from build123d import *

# Parameters (mm, degrees)
SKETCH1_W                    = 16
SKETCH1_H                    = 15
BOSS_EXTRUDE1_DEPTH          = 0.64
EDGE_FLANGE1_STRIP_W         = 5.12
EDGE_FLANGE1_STRIP_H         = 0.64
EDGE_FLANGE1_STRIP_CUT_DEPTH = 16
EDGE_FLANGE1_DEPTH           = 16
SKETCH9_R                    = 1.9
CUT_EXTRUDE1_DEPTH           = 27.570660511
SKETCH10_R                   = 1.9
CUT_EXTRUDE2_DEPTH           = 27.570660511
CHAMFER1_SIZE                = 5
FILLET1_R                    = 2.5


# Sheet-metal steps are written as plain solids
with BuildPart() as part:
    # Sketch1 → Boss-Extrude1 (new body)
    with BuildSketch(Plane(origin=(0, 0, 0), x_dir=(0, 0, -1), z_dir=(1, 0, 0))):
        with Locations((8, 7.5)):
            Rectangle(SKETCH1_W, SKETCH1_H)
    extrude(amount=BOSS_EXTRUDE1_DEPTH)

    # Edge-Flange1 strip (across the edge) → Edge-Flange1 strip cut (cut)
    with BuildSketch(Plane(origin=(0.64, 15, -16), x_dir=(0, -1, 0), z_dir=(0, 0, 1))):
        with Locations((-0.64, -0.32)):
            Rectangle(EDGE_FLANGE1_STRIP_W, EDGE_FLANGE1_STRIP_H)
    extrude(amount=EDGE_FLANGE1_STRIP_CUT_DEPTH, mode=Mode.SUBTRACT)

    # Edge-Flange1 section (across the edge) → Edge-Flange1 (add)
    with BuildSketch(Plane(origin=(0.64, 15, -16), x_dir=(0, -1, 0), z_dir=(0, 0, 1))):
        with BuildLine():
            Line((0, 1.28), (0, 14.36))
            Line((0, 14.36), (0.64, 14.36))
            Line((0.64, 14.36), (0.64, 1.28))
            ThreePointArc((0.64, 1.28), (1.01490332, 0.37490332), (1.92, 0))
            Line((1.92, 0), (1.92, -0.64))
            ThreePointArc((1.92, -0.64), (0.56235498, -0.07764502), (0, 1.28))
        make_face()
    extrude(amount=EDGE_FLANGE1_DEPTH)

    # Sketch9 → Cut-Extrude1 (cut, through all)
    with BuildSketch(Plane.ZY):
        with Locations((-12, 5)):
            Circle(SKETCH9_R)
        with Locations((-4, 5)):
            Circle(SKETCH9_R)
    extrude(amount=-CUT_EXTRUDE1_DEPTH, mode=Mode.SUBTRACT)

    # Sketch10 → Cut-Extrude2 (cut, through all)
    with BuildSketch(Plane(origin=(0, 15, 0), x_dir=(1, 0, 0), z_dir=(0, 1, 0))):
        with Locations(Location((10, 8, 0), (0, 0, 180))):
            Circle(SKETCH10_R)
    extrude(amount=-CUT_EXTRUDE2_DEPTH, mode=Mode.SUBTRACT)

    # Chamfer1
    chamfer1_edges = [part.edges().sort_by_distance(p)[0] for p in [
        (15, 14.68, -16),
        (15, 14.68, 0),
    ]]
    chamfer(chamfer1_edges, length=CHAMFER1_SIZE)

    # Fillet1
    fillet1_edges = [part.edges().sort_by_distance(p)[0] for p in [
        (10, 14.68, -16),
        (15, 14.68, -5),
        (15, 14.68, -11),
        (10, 14.68, 0),
        (0.32, 0, 0),
        (0.32, 0, -16),
    ]]
    fillet(fillet1_edges, radius=FILLET1_R)


solid = part.part
Read the model definition and answer for the solid it produces. Units are mm, in the model's axes. A direction names the side the tool comes from. Coordinates: 2 decimals unless noted, no trailing zeros. Loops run counter-clockwise (first coordinate to the right, second up) from the corner with the lowest first, then second, coordinate; pieces in that order, holes last. Notation, with made-up numbers: (21.25, 9.5) -> (36.25, 9.5) arc R17 ccw to (36.25, 39.5) -> close; hole circle Ø7 at (0.25, 2). An arc over 180 degrees is marked (long way). Write item = value, one per line. Start each with the question number.
1) The part is cut by section B-B, the plane z = -12. Determine the outline of the cut face in (x, y), plus the area to 3 significant figures.
2) The part is cut by section D-D, the plane z = -1.75. Determine the outline of the cut face in (x, y).
3) Given P1, Ø5, axis at y = 9, z = -5, coming from the -X side; P2, Ø4, axis at y = 4.5, z = -10, coming from the +X side; P3, Ø6, axis at x = 9, z = -14, coming from the -Y side, each flat-ended and moving along its own axis, determine where each tip first touches the part or whether it passes through.
4) The part is cut by section C-C, the plane x = 8.75. Determine the outline of the cut face in (y, z), plus the area to 3 significant figures.
5) For faces 5 (the face through (0.64, 7, -8)), 6 (the face through (0.2, 10.6, 0)), determine the directions among +Z, -Z, +X, -X, +Y, -Y from which every point of the face is accessible in a straight line to the end or side of a thin tool.
6) The part is cut by section A-A, the plane y = 5. Determine the outline of the cut face in (x, z).
7) Find the intervals of material crossed by L1, parallel to Y at x = 2.25, z = -15; L2, parallel to X at y = 12.5, z = -8; L3, parallel to Y at x = 0.3, z = -4, in increasing order. Write a range as from..to.
8) The mould has two halves that part along Y. Classify faces 1 (the face through (0.316, 6.284, -5.4)), 2 (the face through (0.324, 0.752, -15.287)), 3 (the face through (0.316, 6.602, -10.979)), 4 (the face through (0.2, 10.6, -16)): pulls with the +Y half, pulls with the -Y half, needs draft (parallel to the pull), parting line crosses it, or undercut.
Result:
q1.outline = (0, 0) -> (0.64, 0) -> (0.64, 3.1) -> (0, 3.1) -> close; (0, 6.9) -> (0.64, 6.9) -> (0.64, 13.08) arc R1.28 cw to (1.92, 14.36) -> (14, 14.36) -> (14, 15) -> (1.92, 15) arc R1.92 ccw to (0, 13.08) -> close
q1.area = 15.3 mm²
q2.outline = (0, 0.12) -> (0.64, 0.12) -> (0.64, 13.08) arc R1.28 cw to (1.92, 14.36) -> (11.75, 14.36) -> (11.75, 15) -> (1.92, 15) arc R1.92 ccw to (0, 13.08) -> close
q3.P1 = 0
q3.P2 = 0.64
q3.P3 = 14.36
q4.outline = (14.36, -16) -> (15, -16) -> (15, -9.43) -> (14.36, -9.43) -> close; (14.36, -6.57) -> (15, -6.57) -> (15, 0) -> (14.36, 0) -> close
q4.area = 8.41 mm²
q5.face_5 = +Z, -Z, +X, -Y
q5.face_6 = +Z, +X, -X, +Y, -Y
q6.outline = (0, -16) -> (0.64, -16) -> (0.64, -13.9) -> (0, -13.9) -> close; (0, -10.1) -> (0.64, -10.1) -> (0.64, -5.9) -> (0, -5.9) -> close; (0, -2.1) -> (0.64, -2.1) -> (0.64, 0) -> (0, 0) -> close
q7.L1 = 14.36..15
q7.L2 = 0..0.64
q7.L3 = 0..3.1, 6.9..14.11
q8.face_1 = undercut
q8.face_2 = pulls with the -Y half
q8.face_3 = undercut
q8.face_4 = needs draft
